Geometry: see drawing. Coordinates: mm, zero at the bounding-box minimum. Give positions to 0.01 mm unless a question says otherwise; leave off trailing zeros. Order: outer loops, then holes, each group sorted by start corner. A loop starts at its lowest first (then second) coordinate and runs counter-clockwise, first axis right, second up. Notation, with made-up numbers: M 36,-36.5 L 50,-36.5 A24 cw 50,-7.5 Z; hole C -17.75,33 d3. An arc over 180 degrees is marked long. Answer as a JSON object with one key per item and string values. Group by question number.
1. Section query B-B (y = 1.8). Output: boundary loops of the cut face in (x, z).
2. Section query C-C (x = 16). Output: boundary loops of the cut face in (y, z).
3. Material intervals for L1, parallel to X at y = 0.45, z = 6.7; L2, parallel to Z at x = 7.5, y = 1.75; L3, parallel to X at y = 0.7, z = 6 (1 decimal), sorted ascending. Write a range as [from, to].
4. Section query A-A (x = 20). Output: boundary loops of the cut face in (y, z).
5. Pin query (flat end, axial travel): P1, Ø4.5, axis at x = 13, z = 6.5, coming from the +Y side; P2, Ø2, axis at y = 1.8, z = 1.8, coming from the +X side; P3, Ø1.2, axis at x = 20, z = 6.7, coming from the -Y side; P4, Ø1.8, axis at y = 2.5, z = 2, coming from the -X side. Return the tip coordinate at first contact, or that it passes through.
6. Section query D-D (z = 8). Output: boundary loops of the cut face in (x, y).
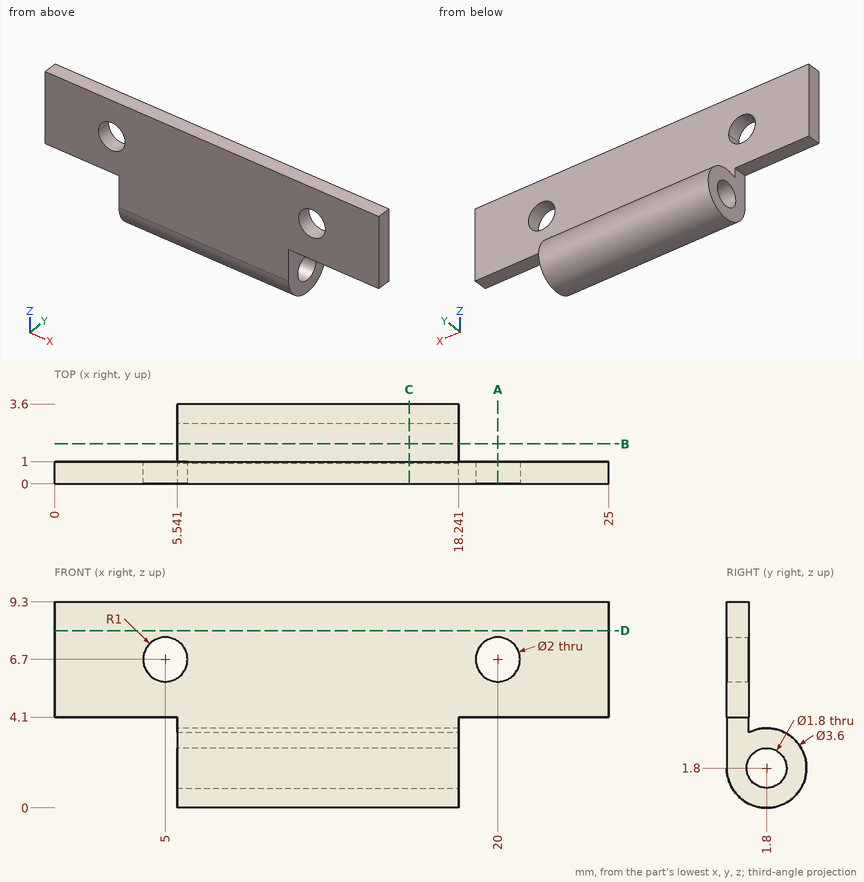
Answer sheet:
{
 "1": {"outline": "M 5.54,0 L 18.24,0 L 18.24,0.9 L 5.54,0.9 Z; M 5.54,2.7 L 18.24,2.7 L 18.24,3.6 L 5.54,3.6 Z"},
 "2": {"outline": "M 0,1.8 A1.8 ccw long 1,3.41 L 1,9.3 L 0,9.3 Z; hole C 1.8,1.8 d1.8"},
 "3": {"L1": "[0, 4], [6, 19], [21, 25]", "L2": "[0, 0.9], [2.7, 3.6]", "L3": "[0, 4.3], [5.7, 19.3], [20.7, 25]"},
 "4": {"outline": "M 0,4.1 L 1,4.1 L 1,5.7 L 0,5.7 Z; M 0,7.7 L 1,7.7 L 1,9.3 L 0,9.3 Z"},
 "5": {"P1": "y = 1", "P2": "x = 18.24", "P3": "through", "P4": "x = 5.54"},
 "6": {"outline": "M 0,0 L 25,0 L 25,1 L 0,1 Z"}
}
